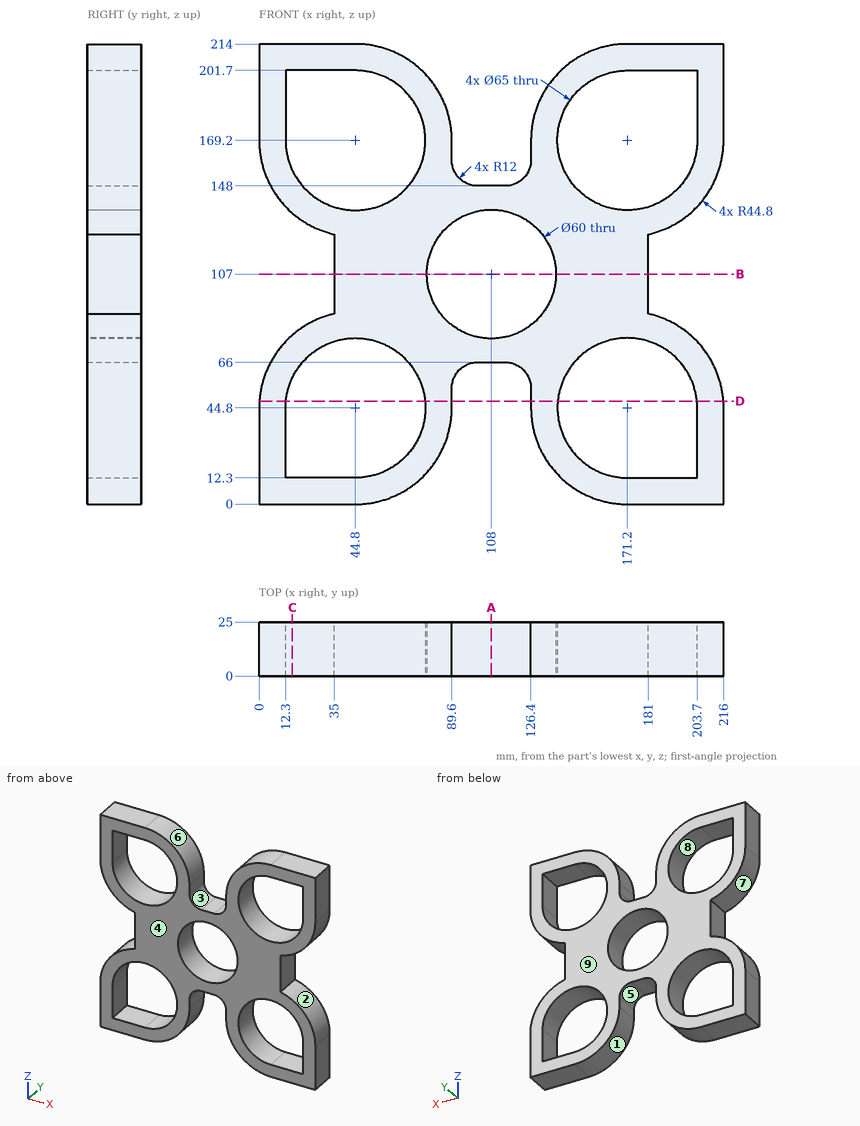
Verification items for this drawing (mm, ordinates from the low corner). A direction names the side the tool comes from. Round coordinates to 2 decimals unless told otherwise and drop trailing zeros. Order: outer loops, then holes, each group sorted by start corner. A loop starts at its lowest first (then second) coordinate and runs counter-clockwise, first axis right, second up. Notation, with made-up numbers: (55, 38) - (107, 38) arc R15 ccw to (107, 62) - close; hole circle Ø6 at (-8.5, -7.75). An arc over 180 degrees is marked (long way). Use CSV: the item, a comma, the result in double quotes.
(1) Gauge pin test, flat ends, axial feed: pin 1 Ø7.5 at (y, z) = (12, 109.5) entering from +X; pin 2 Ø8 at (y, z) = (6, 137.5) entering from +X; pin 3 Ø5 at (y, z) = (11.5, 68) entering from +X. Record the tip position at first contact, or that the pin passes through.
Entries:
pin 1,"x = 181"
pin 2,"x = 206.41"
pin 3,"x = 210.93"
(2) Section check C-C on x = 15.5. Record the boundary of the cut face in (y, z), and give its area (3 significant figures).
Entries:
outline,"(0, 0) - (25, 0) - (25, 12.3) - (0, 12.3) - close; (0, 58.86) - (25, 58.86) - (25, 78.69) - (0, 78.69) - close; (0, 135.31) - (25, 135.31) - (25, 155.14) - (0, 155.14) - close; (0, 201.7) - (25, 201.7) - (25, 214) - (0, 214) - close"
area,"1,610 mm^2"
(3) Section check D-D on z = 48. Record the boundary of the cut face in (x, y), and give its area (3 significant figures).
Entries:
outline,"(0.11, 0) - (12.46, 0) - (12.46, 25) - (0.11, 25) - close; (77.14, 0) - (89.6, 0) - (89.6, 25) - (77.14, 25) - close; (126.4, 0) - (138.86, 0) - (138.86, 25) - (126.4, 25) - close; (203.54, 0) - (215.89, 0) - (215.89, 25) - (203.54, 25) - close"
area,"1,240 mm^2"
(4) Thickness scan on probe 1 along X at (y, z) = (9, 169.2); probe 2 along Z at (x, y) = (171.2, 9); probe 3 along X at (y, z) = (10, 39). Record the ranges inside material, lowest first. Write a range as from..to.
Entries:
probe 1,"0..12.3, 77.3..89.6, 126.4..138.7, 203.7..216"
probe 2,"0..12.3, 77.3..136.7, 201.7..214"
probe 3,"0..12.3, 76.78..89.22, 126.78..139.22, 203.7..216"
(5) Section check B-B on z = 107. Record the boundary of the cut face in (x, y), and give its area (3 significant figures).
Entries:
outline,"(35, 0) - (78, 0) - (78, 25) - (35, 25) - close; (138, 0) - (181, 0) - (181, 25) - (138, 25) - close"
area,"2,150 mm^2"
(6) Access from +Z, -Z, +X, -X, +Y, -Y to the whole of each face (thin tool, end or side, straight path). Record for the marked faces 5, 6, 7, 8 and 9.
Entries:
face 5,"-Z, +Y, -Y"
face 6,"+Z, +Y, -Y"
face 7,"-X, +Y, -Y"
face 8,"+Y, -Y"
face 9,"+Z, -Z, +X, -X, +Y"
(7) Mould release check, pull along Z, two halves, no side actions. Record for the marked faces 1, 2, 3 and 4: released by +Z, released by -Z, zero draft, split by the parting line, or undercut.
Entries:
face 1,"released by -Z"
face 2,"undercut"
face 3,"released by +Z"
face 4,"zero draft"
(8) Section check A-A on x = 108. Record the boundary of the cut face in (y, z).
Entries:
outline,"(0, 66) - (25, 66) - (25, 77) - (0, 77) - close; (0, 137) - (25, 137) - (25, 148) - (0, 148) - close"
